Can you work these out from the model? Positions are in its coordinate system, mm. Face numbers are marked on the shaded views. A direction names the side the tool comes from. Coordinates: 2 decimals unless noted, no trailing zeros. Loops run counter-clockwise (first coordinate to the right, second up) from the corner with the lowest first, then second, coordinate; pieces in that order, holes last.
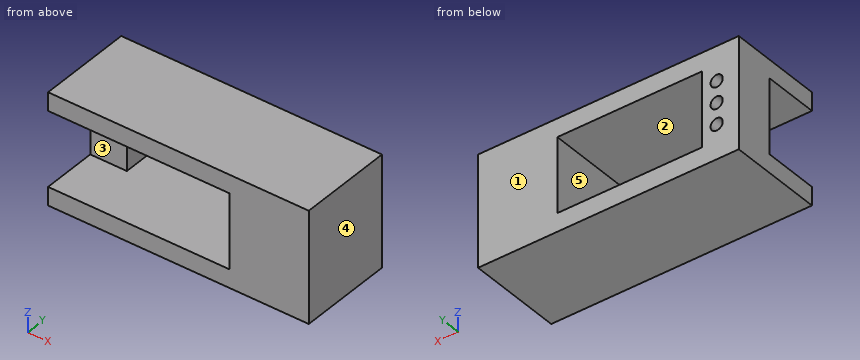
```python
from build123d import *

# Parameters (mm, degrees)
SKETCH1_W           = 23.75
SKETCH1_H           = 12.25
BOSS_EXTRUDE1_DEPTH = 15.6
SKETCH2_W           = 12.25
SKETCH2_H           = 9
CUT_EXTRUDE1_DEPTH  = 10
SKETCH3_R           = 1
CUT_EXTRUDE2_DEPTH  = 3


with BuildPart() as part:
    # Sketch1 → Boss-Extrude1 (new body)
    with BuildSketch(Plane(origin=(0, 0, 0), x_dir=(1, 0, 0), z_dir=(0, 1, 0))):
        Polygon((17.875, -9.125), (24.875, -9.125), (24.875, 9.125), (17.875, 9.125), (-17.875, 9.125), (-17.875, -9.125), align=None)
        Rectangle(SKETCH1_W, SKETCH1_H, mode=Mode.SUBTRACT)
    extrude(amount=BOSS_EXTRUDE1_DEPTH)

    # Sketch2 → Cut-Extrude1 (cut)
    with BuildSketch(Plane.ZY.offset(17.875)):
        with Locations((0, 4.5)):
            Rectangle(SKETCH2_W, SKETCH2_H)
    extrude(amount=-CUT_EXTRUDE1_DEPTH, mode=Mode.SUBTRACT)

    # Sketch3 → Cut-Extrude2 (cut)
    with BuildSketch(Plane(origin=(0, 15.6, 0), x_dir=(1, 0, 0), z_dir=(0, 1, 0))):
        with Locations(Location((-14.245, 3.495, 0), (0, 0, 270))):
            Circle(SKETCH3_R)
        with Locations(Location((-14.245, -0.005, 0), (0, 0, 270))):
            Circle(SKETCH3_R)
        with Locations(Location((-14.245, -3.505, 0), (0, 0, 270))):
            Circle(SKETCH3_R)
    extrude(amount=-CUT_EXTRUDE2_DEPTH, mode=Mode.SUBTRACT)


solid = part.part
```
Item 1: Suppose I cut it at A-A, the plane x = 10.5. Please give me the cut outline in (y, z) (3 decimals), plus the area to 3 significant figures.
Results are:
outline: (0, -9.125) - (15.6, -9.125) - (15.6, -6.125) - (0, -6.125) - close; (0, 6.125) - (15.6, 6.125) - (15.6, 9.125) - (0, 9.125) - close
area: 93.6 mm2
Item 2: Suppose I cut it at B-B, the plane z = 1.5. Please give me the cut outline in (x, y) (3 decimals).
Results are:
outline: (-17.875, 9) - (-11.875, 9) - (-11.875, 15.6) - (-17.875, 15.6) - close; (11.875, 0) - (24.875, 0) - (24.875, 15.6) - (11.875, 15.6) - close
Item 3: I'm going to push flat-ended pins straight in: P1, Ø1, axis at x = -14.5, z = -3.5, coming from the +Y side; P2, Ø1.8, axis at x = -14.245, z = 3.505, coming from the -Y side. Where does each tip first touch, or does it pass through?
Results are:
P1: stops at y = 12.6
P2: stops at y = 9
Item 4: We'd pull the mould along X, two halves only. Please class the marked faces 3, 4 and 5: +X half, -X half, draft (parallel to the pull), parting line (faces both ways), or undercut.
Results are:
face 3: draft
face 4: +X half
face 5: undercut
Item 5: Suppose I cut it at D-D, the plane y = 3. Please give me the cut outline in (x, z) (3 decimals).
Results are:
outline: (-17.875, -9.125) - (24.875, -9.125) - (24.875, 9.125) - (-17.875, 9.125) - (-17.875, 6.125) - (11.875, 6.125) - (11.875, -6.125) - (-17.875, -6.125) - close
Item 6: On a 3-axis mill with a long thin cutter (end or side, diameter ignored), from which of +Z, -Z, +X, -X, +Y, -Y can I reach the whole of each face in a straight line? I mean the marked faces 1 and 2. Say none if no direction works.
Results are:
face 1: +Z, -Z, +X, -X, +Y
face 2: -Y
Item 7: Suppose I cut it at C-C, the plane y = 12. Please give me the cut outline in (x, z) (3 decimals).
Results are:
outline: (-17.875, -9.125) - (24.875, -9.125) - (24.875, 9.125) - (-17.875, 9.125) - close; hole (-11.875, -6.125) - (11.875, -6.125) - (11.875, 6.125) - (-11.875, 6.125) - close
Item 8: I need wall thicknesses on line 1 along X through (y, z) = (13, 3.5) (3 decimals); line 2 along Z through (x, y) = (-10, 13) (3 decimals); line 3 along X through (y, z) = (13.25, 5) (3 decimals). Which ranges of each line are inside material? Lowest first, please.
Results are:
line 1: x = -17.875 to -15.245, -13.245 to -11.875, 11.875 to 24.875
line 2: z = -9.125 to -6.125, 6.125 to 9.125
line 3: x = -17.875 to -11.875, 11.875 to 24.875
